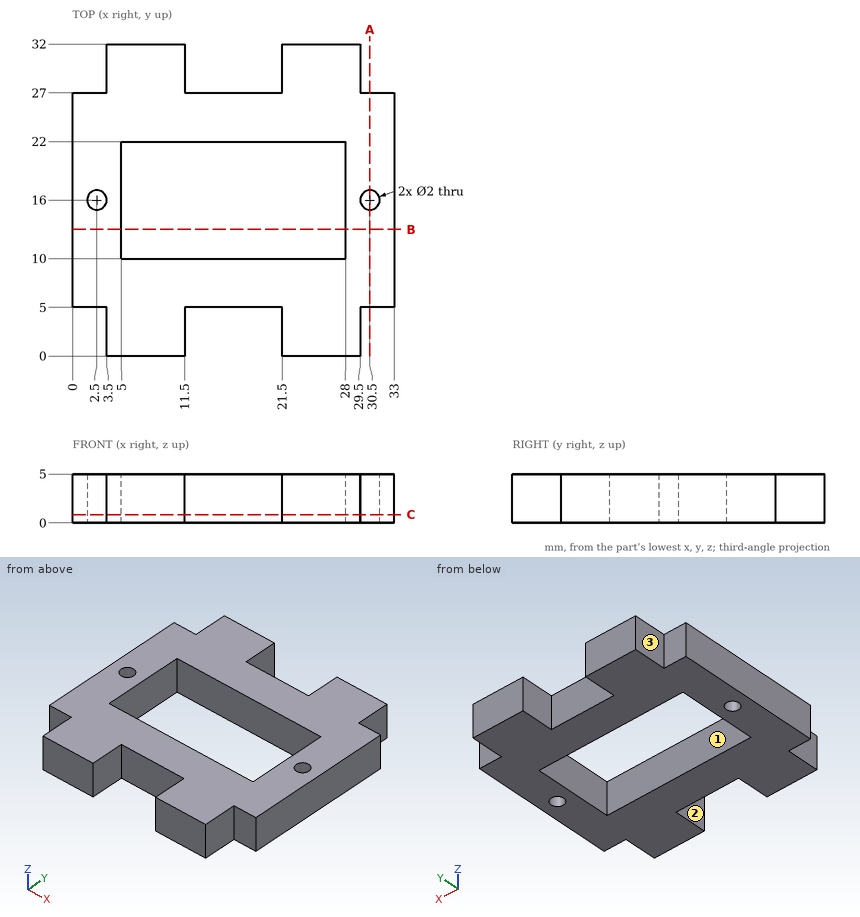
The drawing under review shows one solid part. Ordinate dimensions are in mm from its lowest x, y, z. A direction names the side the tool comes from. Give positions to 0.01 mm unless a question says otherwise; leave off trailing zeros. Write each loop counter-clockwise with the first axis right and the second up, starting at its lowest first coordinate (ties: lowest second). Pieces come first, ordered by that corner, then holes.
1. Add section B-B, the plane y = 13. Write out the cut boundary in (x, z).
2. Add section C-C, the plane z = 0.85. Write out the cut boundary in (x, y).
3. Add section A-A, the plane x = 30.5. Write out the cut boundary in (y, z).
4. Tool access review of the marked faces 1, 2 and 3: name each direction out of +Z, -Z, +X, -X, +Y, -Y from which nothing blocks a thin tool from reaching the whole face with its end or side.
5. For P1, Ø10, axis at x = 10, y = 21, coming from the -Z side; P2, Ø2, axis at x = 15.5, z = 2.5, coming from the +Y side; P3, Ø1.8, axis at x = 32, z = 2, coming from the -Y side; P4, Ø2.5, axis at y = 2.5, z = 2.5, coming from the +X side, all flat-tipped, find the tip position at first contact; note any pin that passes through.
6. Wall thickness on L1, parallel to X at y = 14.5, z = 1.65; L2, parallel to Y at x = 30.5, z = 3.2; L3, parallel to Y at x = 21, z = 0.25: over which ranges is each line inside the solid? List them lowest first.
Worked answers:
1. outline: (0, 0) - (5, 0) - (5, 5) - (0, 5) - close; (28, 0) - (33, 0) - (33, 5) - (28, 5) - close
2. outline: (0, 5) - (3.5, 5) - (3.5, 0) - (11.5, 0) - (11.5, 5) - (21.5, 5) - (21.5, 0) - (29.5, 0) - (29.5, 5) - (33, 5) - (33, 27) - (29.5, 27) - (29.5, 32) - (21.5, 32) - (21.5, 27) - (11.5, 27) - (11.5, 32) - (3.5, 32) - (3.5, 27) - (0, 27) - close; hole circle Ø2 at (2.5, 16); hole (5, 10) - (28, 10) - (28, 22) - (5, 22) - close; hole circle Ø2 at (30.5, 16)
3. outline: (5, 0) - (15, 0) - (15, 5) - (5, 5) - close; (17, 0) - (27, 0) - (27, 5) - (17, 5) - close
4. face 1: +Z, -Z
4. face 2: +Z, -Z, -Y
4. face 3: +Z, -Z, -X, +Y
5. P1: stops at z = 0
5. P2: stops at y = 27
5. P3: stops at y = 5
5. P4: stops at x = 29.5
6. L1: x = 0 to 5, 28 to 33
6. L2: y = 5 to 15, 17 to 27
6. L3: y = 5 to 10, 22 to 27
